from build123d import *

# Parameters (mm, degrees)
BOSS_EXTRUDE1_DEPTH      = 2.7432
BOSS_EXTRUDE1_DEPTH_BACK = 2.7432
CUT_EXTRUDE1_DEPTH       = 2.794
CUT_EXTRUDE1_DEPTH_BACK  = 2.794
CUT_EXTRUDE2_DEPTH       = 2.794
CUT_EXTRUDE2_DEPTH_BACK  = 2.794


with BuildPart() as part:
    # Sketch1 → Boss-Extrude1 (new, two sides: drawn at the far end of the back side and taken through both)
    with BuildSketch(Plane(origin=(0, 0, 0), x_dir=(0, 0, -1), z_dir=(1, 0, 0)).offset(-BOSS_EXTRUDE1_DEPTH_BACK)):
        Polygon((-0.8382, -1.8034), (-0.7366, -1.905), (-0.5334, -1.905), (-0.4318, -1.8034), (-0.4318, 1.016), (0.4318, 1.016), (0.4318, -1.8034), (0.5334, -1.905), (0.7366, -1.905), (0.8382, -1.8034), (0.8382, 4.5974), (0.7366, 4.699), (0.5334, 4.699), (0.4318, 4.5974), (0.4318, 1.4224), (-0.4318, 1.4224), (-0.4318, 4.5974), (-0.5334, 4.699), (-0.7366, 4.699), (-0.8382, 4.5974), align=None)
    extrude(amount=BOSS_EXTRUDE1_DEPTH + BOSS_EXTRUDE1_DEPTH_BACK)

    # Sketch2 → Cut-Extrude1 (cut, two sides: drawn at the far end of the back side and taken through both)
    with BuildSketch(Plane.XY.offset(-CUT_EXTRUDE1_DEPTH_BACK)):
        Polygon((-3.6068, -2.413), (4.0132, -2.413), (4.0132, -1.905), (3.6068, -1.905), (3.6068, 1.016), (2.7432, 1.016), (2.7432, -1.905), (2.3368, -1.905), (2.3368, 1.016), (1.4732, 1.016), (1.4732, -1.905), (1.0668, -1.905), (1.0668, 1.016), (0.2032, 1.016), (0.2032, -1.905), (-0.2032, -1.905), (-0.2032, 1.016), (-1.0668, 1.016), (-1.0668, -1.905), (-1.4732, -1.905), (-1.4732, 1.016), (-2.3368, 1.016), (-2.3368, -1.905), (-2.7432, -1.905), (-2.7432, 1.016), (-3.6068, 1.016), align=None)
    extrude(amount=CUT_EXTRUDE1_DEPTH + CUT_EXTRUDE1_DEPTH_BACK, mode=Mode.SUBTRACT)

    # Sketch3 → Cut-Extrude2 (cut, two sides: drawn at the far end of the back side and taken through both)
    with BuildSketch(Plane.XY.offset(-CUT_EXTRUDE2_DEPTH_BACK)):
        Polygon((-3.6068, 5.3594), (-3.6068, 1.4224), (-2.7432, 1.4224), (-2.7432, 4.8514), (-2.3368, 4.8514), (-2.3368, 1.4224), (-1.4732, 1.4224), (-1.4732, 4.8514), (-1.0668, 4.8514), (-1.0668, 1.4224), (-0.2032, 1.4224), (-0.2032, 4.8514), (0.2032, 4.8514), (0.2032, 1.4224), (1.0668, 1.4224), (1.0668, 4.8514), (1.4732, 4.8514), (1.4732, 1.4224), (2.3368, 1.4224), (2.3368, 4.8514), (2.7432, 4.8514), (2.7432, 1.4224), (3.6068, 1.4224), (3.6068, 4.8514), (4.0132, 4.8514), (4.0132, 5.3594), align=None)
    extrude(amount=CUT_EXTRUDE2_DEPTH + CUT_EXTRUDE2_DEPTH_BACK, mode=Mode.SUBTRACT)


solid = part.part
Check sheet for the modelled part. Datum: model origin and axes. Units: mm. Round coordinates to 2 decimals unless told otherwise and drop trailing zeros. Loops run counter-clockwise (first coordinate to the right, second up) from the corner with the lowest first, then second, coordinate; pieces in that order, holes last. Notation, with made-up numbers: M 54,31 L 110,31 A30 ccw 110,55 Z; hole C 57.5,69.5 d5. An arc over 180 degrees is marked long. One line per item, written item: value.
(1) Thickness scan on line 1 (X direction, y = -1, z = -0.5); line 2 (Z direction, x = 1.4, y = -1); line 3 (Y direction, x = 0.5, z = -0.35). Record the ranges inside material, lowest first.
Computed values:
line 1: x = -2.74 to -2.34, -1.47 to -1.07, -0.2 to 0.2, 1.07 to 1.47, 2.34 to 2.74
line 2: z = -0.84 to -0.43, 0.43 to 0.84
line 3: y = 1.02 to 1.42
(2) Sectioned sample at A-A, the plane x = 0.1. Record the cut outline in (y, z) (3 decimals), then the cut area to 3 significant figures.
Computed values:
outline: M -1.905,-0.737 L -1.803,-0.838 L 4.597,-0.838 L 4.699,-0.737 L 4.699,-0.533 L 4.597,-0.432 L 1.422,-0.432 L 1.422,0.432 L 4.597,0.432 L 4.699,0.533 L 4.699,0.737 L 4.597,0.838 L -1.803,0.838 L -1.905,0.737 L -1.905,0.533 L -1.803,0.432 L 1.016,0.432 L 1.016,-0.432 L -1.803,-0.432 L -1.905,-0.533 Z
area: 5.68 mm^2
(3) Release check for a two-part mould opening along X. For faces 1 (the face through (0, 1, -0.838)), 2 (the face through (0, 1.016, 0)), 3 (the face through (2.743, 1.4, 0.6)) record: +X half, -X half, draft (parallel to the pull), parting line (faces both ways), or undercut.
Computed values:
face 1: draft
face 2: undercut
face 3: +X half
(4) Sectioned sample at C-C, the plane z = 0.3. Record the cut outline in (x, y), then the cut area to 3 significant figures.
Computed values:
outline: M -2.74,1.02 L 2.74,1.02 L 2.74,1.42 L -2.74,1.42 Z
area: 2.23 mm^2
(5) Sectioned sample at B-B, the plane y = 3. Count the separate pieces of the cut face and the enclosed holes in it, then the cut area to 3 significant figures.
Computed values:
separate pieces: 10
enclosed holes: 0
area: 1.65 mm^2
(6) Sectioned sample at D-D, the plane x = 2.2. Record the cut outline in (y, z), then the cut area to 3 significant figures.
Computed values:
outline: M 1.02,-0.84 L 1.42,-0.84 L 1.42,0.84 L 1.02,0.84 Z
area: 0.681 mm^2
